from build123d import *

# Parameters (mm, degrees)
SKETCH1_R           = 14.25
SKETCH1_R_2         = 11.25
BOSS_EXTRUDE1_DEPTH = 24
SKETCH2_R           = 13.8
SKETCH2_R_2         = 2.25
BOSS_EXTRUDE2_DEPTH = 4
FILLET1_R           = 1
CUT_EXTRUDE1_DEPTH  = 9


with BuildPart() as part:
    # Sketch1 → Boss-Extrude1 (new body)
    with BuildSketch(Plane(origin=(0, 0, 0), x_dir=(1, 0, 0), z_dir=(0, 1, 0))):
        Circle(SKETCH1_R)
        Circle(SKETCH1_R_2, mode=Mode.SUBTRACT)
    extrude(amount=BOSS_EXTRUDE1_DEPTH)

    # Sketch2 → Boss-Extrude2 (add)
    with BuildSketch(Plane(origin=(0, 24, 0), x_dir=(1, 0, 0), z_dir=(0, 1, 0))):
        Circle(SKETCH2_R)
        Circle(SKETCH2_R_2, mode=Mode.SUBTRACT)
    extrude(amount=BOSS_EXTRUDE2_DEPTH)

    # Fillet1
    fillet1_edges = [part.edges().sort_by_distance(p)[0] for p in [
        (-11.25, 0, 0),
    ]]
    fillet(fillet1_edges, radius=FILLET1_R)

    # Sketch3 → Cut-Extrude1 (cut)
    with BuildSketch(Plane.XZ):
        with BuildLine():
            Line((2, 14.25), (2, -14.25))
            ThreePointArc((2, -14.25), (0, -16.25), (-2, -14.25))
            Line((-2, -14.25), (-2, 14.25))
            ThreePointArc((-2, 14.25), (0, 16.25), (2, 14.25))
        make_face()
    extrude(amount=-CUT_EXTRUDE1_DEPTH, mode=Mode.SUBTRACT)


solid = part.part
Work out the finished part from the listing and answer in its coordinate system (mm). A direction names the side the tool comes from. Give positions to 0.01 mm unless a question says otherwise; leave off trailing zeros. Order: outer loops, then holes, each group sorted by start corner. A loop starts at its lowest first (then second) coordinate and runs counter-clockwise, first axis right, second up. Notation, with made-up numbers: M -37,28 L -23,28 A35 cw -23,65 Z; hole C 46.25,39 d3. An arc over 180 degrees is marked long. Return JSON: item names as keys, results as strings.
Q1. Find section A-A, the plane z = 0. Write down the section's boundary in (x, y), and give its area (3 significant figures).
Answer below:
{"outline": "M -14.25,0 L -12.25,0 A1 ccw -11.25,1 L -11.25,24 L -2.25,24 L -2.25,28 L -13.8,28 L -13.8,24 L -14.25,24 Z; M 2.25,24 L 11.25,24 L 11.25,1 A1 ccw 12.25,0 L 14.25,0 L 14.25,24 L 13.8,24 L 13.8,28 L 2.25,28 Z", "area": "236 mm^2"}
Q2. Find section D-D, the plane y = 10.75. Write down the section's boundary in (x, z).
Answer below:
{"outline": "C 0,0 d28.5; hole C 0,0 d22.5"}
Q3. Find section C-C, the plane y = 2.75. Write down the section's boundary in (x, z).
Answer below:
{"outline": "M -2,-14.11 L -2,-11.07 A11.25 cw -2,11.07 L -2,14.11 A14.25 ccw Z; M 2,-14.11 A14.25 ccw 2,14.11 L 2,11.07 A11.25 cw 2,-11.07 Z"}
Q4. Each of these flat-tipped pins is pushed along its axis until it touches: pin 1 (3.5 mm diameter, centred on y = 4.5, z = 13, fed in from +X); pin 2 (12 mm diameter, centred on x = -7, y = 5, fed in from -Z); pin 3 (5 mm diameter, centred on y = 5, z = -4.5, fed in from -X); pin 4 (6 mm diameter, centred on y = 8, z = 1, fed in from -X). Where does it stop, or does it pass through?
Answer below:
{"pin 1": "stops at x = 8.75", "pin 2": "stops at z = -14.11", "pin 3": "stops at x = -14.11", "pin 4": "stops at x = -14.25"}
Q5. Which of the six approach directions +Z, -Z, +X, -X, +Y, -Y give full straight-line access (tool end or side, diameter ignored) to faces 4 (the face through (-14, 24, -1)), 5 (the face through (-2.439, 12.339, 10.982)), 6 (the face through (2, 4, 13))?
Answer below:
{"face 4": "+Y", "face 5": "-Y", "face 6": "+Z, -Z, -Y"}
Q6. The mould has two halves that part along X. Classify faces 1 (the face through (-3.09, 11.83, 13.91)), 2 (the face through (2, 4, -13)), 3 (the face through (13, 0, 0)): pulls with the +X half, pulls with the -X half, needs draft (parallel to the pull), parting line crosses it, or undercut.
Answer below:
{"face 1": "parting line crosses it", "face 2": "undercut", "face 3": "needs draft"}
Q7. Find section B-B, the plane x = 0. Write down the section's boundary in (y, z).
Answer below:
{"outline": "M 9,-14.25 L 24,-14.25 L 24,-13.8 L 28,-13.8 L 28,-2.25 L 24,-2.25 L 24,-11.25 L 9,-11.25 Z; M 9,11.25 L 24,11.25 L 24,2.25 L 28,2.25 L 28,13.8 L 24,13.8 L 24,14.25 L 9,14.25 Z"}
Q8. Find the intervals of material crossed by line 1 along X through (y, z) = (14.25, 0); line 2 along Z through (x, y) = (0, 26.3), in increasing order. Write a range as [from, to].
Answer below:
{"line 1": "x = [-14.25, -11.25], [11.25, 14.25]", "line 2": "z = [-13.8, -2.25], [2.25, 13.8]"}
